Check sheet for the modelled part. Datum: model origin and axes. Units: mm. Give positions to 0.01 mm unless a question says otherwise; leave off trailing zeros. Loops run counter-clockwise (first coordinate to the right, second up) from the corner with the lowest first, then second, coordinate; pieces in that order, holes last. Notation, with made-up numbers: (54.25, 20) -> (60.25, 20) arc R13 ccw to (60.25, 38) -> close; hole circle Ø9 at (52.25, 20). An arc over 180 degrees is marked (long way). Answer as CSV lines item,"result". Start each with the question number.
(1) Material ranges on line 1 (Z direction, x = 0, y = 1.15); line 2 (X direction, y = 2.25, z = -1.75); line 3 (X direction, y = 3.35, z = -2.25), recorded low to high. Write a range as from..to.
(2) Section check B-B on z = -3.25. Enter the section's corners in (x, y), plus the area to 3 significant figures.
(3) Section check A-A on x = -25. Enter the section's corners in (y, z), plus the area to 3 significant figures.
(4) Gauge pin test, flat ends, axial feed: pin 1 Ø14.5 at (x, z) = (0, 0) entering from +Y; pin 2 Ø10 at (x, z) = (25, 0) entering from +Y. Record the tip position at first contact, or that the pin passes through.
(5) Section check C-C on y = 2.55. Enter the section's corners in (x, z), plus the area to 3 significant figures.
from build123d import *

# Parameters (mm, degrees)
SKETCH1_W           = 100
SKETCH1_H           = 30
BOSS_EXTRUDE1_DEPTH = 5


with BuildPart() as part:
    # Sketch1 → Boss-Extrude1 (new body)
    with BuildSketch(Plane(origin=(0, 0, 0), x_dir=(1, 0, 0), z_dir=(0, 1, 0))):
        Rectangle(SKETCH1_W, SKETCH1_H)
        with BuildLine():
            ThreePointArc((31.321653543, 0.599330025), (31.95, 0), (31.321653543, -0.599330025))
            ThreePointArc((31.321653543, -0.599330025), (18.65, 0), (31.321653543, 0.599330025))
        make_face(mode=Mode.SUBTRACT)
        with BuildLine():
            ThreePointArc((6.321653543, 0.599330025), (6.95, 0), (6.321653543, -0.599330025))
            ThreePointArc((6.321653543, -0.599330025), (-6.35, 0), (6.321653543, 0.599330025))
        make_face(mode=Mode.SUBTRACT)
        with BuildLine():
            ThreePointArc((-18.678346457, 0.599330025), (-18.05, 0), (-18.678346457, -0.599330025))
            ThreePointArc((-18.678346457, -0.599330025), (-31.35, 0), (-18.678346457, 0.599330025))
        make_face(mode=Mode.SUBTRACT)
    extrude(amount=BOSS_EXTRUDE1_DEPTH)


solid = part.part
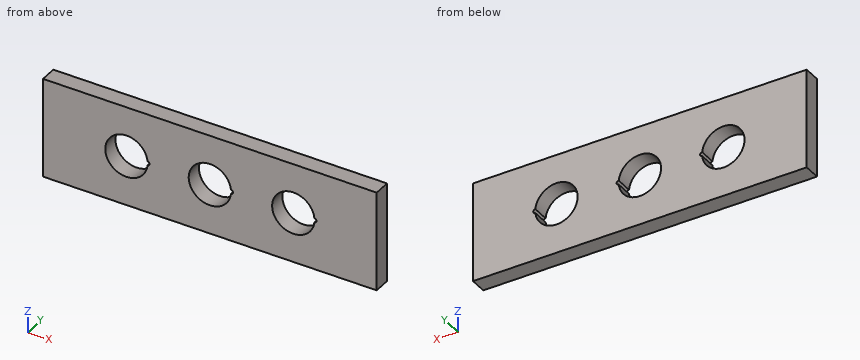
Working result:
1,line 1,"z = -15..-6.35, 6.35..15"
1,line 2,"x = -50..-31.1, -18.9..-6.1, 6.1..18.9, 31.1..50"
1,line 3,"x = -50..-30.94, -19.06..-5.94, 5.94..19.06, 30.94..50"
2,outline,"(-50, 0) -> (-30.46, 0) -> (-30.46, 5) -> (-50, 5) -> close; (-19.54, 0) -> (-5.46, 0) -> (-5.46, 5) -> (-19.54, 5) -> close; (5.46, 0) -> (19.54, 0) -> (19.54, 5) -> (5.46, 5) -> close; (30.46, 0) -> (50, 0) -> (50, 5) -> (30.46, 5) -> close"
2,area,"336 mm^2"
3,outline,"(0, -15) -> (5, -15) -> (5, -6.35) -> (0, -6.35) -> close; (0, 6.35) -> (5, 6.35) -> (5, 15) -> (0, 15) -> close"
3,area,"86.5 mm^2"
4,pin 1,"stops at y = 5"
4,pin 2,"passes through"
5,outline,"(-50, -15) -> (50, -15) -> (50, 15) -> (-50, 15) -> close; hole (-18.68, -0.6) arc R0.6 ccw (long way) to (-18.68, 0.6) arc R6.35 ccw (long way) to start; hole (6.32, -0.6) arc R0.6 ccw (long way) to (6.32, 0.6) arc R6.35 ccw (long way) to start; hole (31.32, -0.6) arc R0.6 ccw (long way) to (31.32, 0.6) arc R6.35 ccw (long way) to start"
5,area,"2,620 mm^2"
